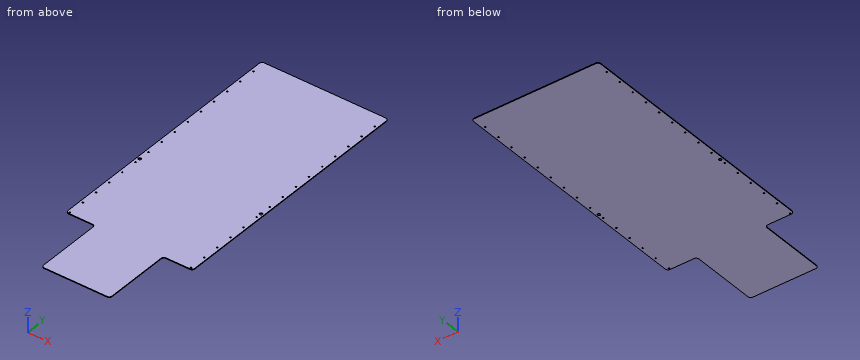
Autodesk Inventor part; units mm, degrees
ref_plane "YZ Plane" through (0, 0, 0) normal (1, 0, 0) x (0, 1, 0)
ref_plane "XZ Plane" through (0, 0, 0) normal (0, 1, 0) x (-1, 0, 0)
ref_plane "XY Plane" through (0, 0, 0) normal (0, 0, 1) x (1, 0, 0)
sketch "Sketch2" plane through (0, 0, 0) normal (0, 0, 1) x (1, 0, 0)
  line L0 (0, 0) -> (566.42, 0)
  line L1 (566.42, 0) -> (566.42, -1727.2)
  line L2 (566.42, -1727.2) -> (0, -1727.2)
  line L3 (0, -1727.2) -> (0, 0)
  dimension "d0" = 566.42
  dimension "d1" = 1727.2
extrude "Extrusion1" add sketch "Sketch2" along normal blind 3.175
sketch "Sketch4" plane through (0, 0, 3.175) normal (0, 0, 1) x (1, 0, 0)
  line L0 (566.42, 0) -> (0, 0)
  line L1 (0, 0) -> (0, -1727.2)
  line L2 (0, -1727.2) -> (566.42, -1727.2)
  line L3 (566.42, -1727.2) -> (566.42, 0)
  line L4 (0, -1727.2) -> (566.42, -1727.2)
  line L5 (68.58, -1727.2) -> (500.38, -1727.2)
  circle A0 centre (68.58, -1391.92) radius 12.7
  circle A1 centre (500.38, -1391.92) radius 12.7
  circle A2 centre (68.58, -1727.2) radius 12.7
  circle A3 centre (500.38, -1727.2) radius 12.7
  dimension "d6" = 25.4
  dimension "d7" = 25.4
  dimension "d8" = 25.4
  dimension "d9" = 25.4
extrude "Extrusion2" add sketch "Sketch4" along normal blind 3.175 contours A0 | A1
sketch "Sketch6" plane through (0, 0, 3.175) normal (0, 0, 1) x (1, 0, 0)
  circle A0 centre (12.7, -1460.5) radius 3.175
  circle A1 centre (553.72, -1460.5) radius 3.175
  circle A2 centre (553.72, -1460.5) radius 4.7625
  circle A3 centre (12.7, -1460.5) radius 4.7625
  point P0 (0, 0)
  dimension "d16" = 9.525
  dimension "d17" = 9.525
extrude "Extrusion4" cut sketch "Sketch6" against normal through all contours A0 | A1 | A2 | A3
sketch "Sketch7" plane through (0, 0, 3.175) normal (0, 0, 1) x (1, 0, 0)
  circle A0 centre (12.7, -1460.5) radius 4.7625
  circle A1 centre (12.7, -1460.5) radius 6.35
  circle A2 centre (553.72, -1460.5) radius 4.7625
  circle A3 centre (553.72, -1460.5) radius 6.35
  point P0 (0, 0)
  dimension "d20" = 12.7
  dimension "d21" = 12.7
extrude "Extrusion5" cut sketch "Sketch7" against normal blind 12.7 contours A3
sketch "Sketch9" plane through (0, 0, 3.175) normal (0, 0, 1) x (1, 0, 0)
  circle A0 centre (553.72, -825.5) radius 6.35
  circle A1 centre (12.7, -825.5) radius 6.35
  circle A2 centre (12.7, -825.5) radius 6.35
  circle A3 centre (553.72, -825.5) radius 6.35
  point P0 (0, 0)
extrude "Extrusion7" cut sketch "Sketch9" against normal blind 3.175
sketch "Sketch10" plane through (0, 0, 3.175) normal (0, 0, 1) x (1, 0, 0)
  line L0 (566.42, 0) -> (566.42, -1727.2)
  line L1 (0, -1732.8892) -> (566.42, -1732.8892)
  line L2 (566.42, -1732.8892) -> (566.42, -1054.0894)
  line L3 (566.42, -1054.0894) -> (0, -1054.0894)
  line L4 (0, -1054.0894) -> (0, -1732.8892)
  point P0 (0, 0)
extrude "Extrusion8" cut sketch "Sketch10" along normal blind 25.4
sketch "Sketch12" plane through (0, 0, 0) normal (0, 0, -1) x (-1, 0, 0)
  line L0 (-133.5248, -1752.8599) -> (-130.3498, -1752.8599)
  line L1 (-130.3498, -1752.8599) -> (-130.3498, -1726.7719)
  line L2 (-130.3498, -1726.7719) -> (-133.5248, -1726.7719)
  line L3 (-133.5248, -1726.7719) -> (-133.5248, -1752.8599)
  line L4 (-133.5248, -1752.8599) -> (-130.3498, -1752.8599)
  line L5 (-133.5248, -1777.5719) -> (-133.5248, -1752.8599)
  line L6 (-82.7248, -1777.5719) -> (-133.5248, -1777.5719)
  line L7 (-82.7248, -1774.3969) -> (-82.7248, -1777.5719)
  line L8 (-130.3498, -1774.3969) -> (-82.7248, -1774.3969)
  line L9 (-130.3498, -1752.8599) -> (-130.3498, -1774.3969)
  line L10 (-130.3498, -1237.6912) -> (0, -1237.6912)
  line L11 (0, -1237.6912) -> (0, -1727.2)
  line L12 (0, -1727.2) -> (-130.3498, -1727.2)
  line L13 (-130.3498, -1727.2) -> (-130.3498, -1237.6912)
  line L14 (0, -1727.2) -> (-566.42, -1727.2)
  line L15 (-566.8989, -1237.6912) -> (-436.5461, -1237.6912)
  line L16 (-436.5461, -1237.6912) -> (-436.5461, -1727.2)
  line L17 (-436.5461, -1727.2) -> (-566.8989, -1727.2)
  line L18 (-566.8989, -1727.2) -> (-566.8989, -1237.6912)
  point P0 (0, 0)
  point P1 (-108.1248, -1263.0912)
  dimension "d32" = 130.3528
extrude "Extrusion9" cut sketch "Sketch12" against normal blind 3.175 contours L1 L13 L10 L11 L12
sketch "Sketch13" plane through (0, 0, 0) normal (0, 0, -1) x (-1, 0, 0)
  line L0 (-566.42, -1727.2) -> (-566.42, 0)
  line L1 (-130.3498, -1727.2) -> (-566.42, -1727.2)
  line L2 (-566.42, -1239.5747) -> (-435.131, -1239.5747)
  line L3 (-435.131, -1239.5747) -> (-435.131, -1727.2)
  line L4 (-435.131, -1727.2) -> (-566.42, -1727.2)
  line L5 (-566.42, -1727.2) -> (-566.42, -1239.5747)
  point P0 (0, 0)
extrude "Extrusion10" cut sketch "Sketch13" against normal blind 3.175
sketch "Sketch14" plane through (0, 0, 0) normal (0, 0, -1) x (-1, 0, 0)
  line L0 (-130.3498, -1727.2) -> (-130.3498, -1237.6912)
  line L1 (-435.131, -1727.2) -> (-130.3498, -1727.2)
  line L2 (-130.3498, -1727.2) -> (-130.3498, -1549.4)
  line L3 (-130.3498, -1549.4) -> (-435.131, -1549.4)
  line L4 (-435.131, -1549.4) -> (-435.131, -1727.2)
  point P0 (0, 0)
  dimension "d35" = 177.8
extrude "Extrusion11" cut sketch "Sketch14" against normal blind 3.175
hole "Hole1" at (12.7, -12.7, 3.175) direction (0, 0, -1) diameter 6.35 depth 12.7 tip angle 118
pattern_linear "Rectangular Pattern1" count 17 spacing 76.2 along (0, -1, 0) of "Hole1"
hole "Hole2" at (553.72, -12.7, 3.175) direction (0, 0, -1) diameter 6.35 depth 12.7 tip angle 118
pattern_linear "Rectangular Pattern2" count 17 spacing 76.2 along (0, -1, 0) of "Hole2"
fillet "Fillet1" radius 12.7 8 edges at (566.42, 0, 1.5875) (0, 0, 1.5875) (566.42, -1239.5747, 1.5875) (435.131, -1239.5747, 1.5875) (435.131, -1549.4, 1.5875) (0, -1237.6912, 1.5875) (130.3498, -1237.6912, 1.5875) (130.3498, -1549.4, 1.5875)
sketch "Sketch15" plane through (0, 0, 3.175) normal (0, 0, 1) x (1, 0, 0)
  arc A0 (130.3498, -1536.7) -> (143.0498, -1549.4) centre (143.0498, -1536.7) ccw
  line L0 (143.0498, -1549.4) -> (422.431, -1549.4)
  arc A1 (422.431, -1549.4) -> (435.131, -1536.7) centre (422.431, -1536.7) ccw
  line L1 (435.131, -1536.7) -> (435.131, -1252.2747)
  arc A2 (447.831, -1239.5747) -> (435.131, -1252.2747) centre (447.831, -1252.2747) ccw
  line L2 (447.831, -1239.5747) -> (553.72, -1239.5747)
  arc A3 (553.72, -1239.5747) -> (566.42, -1226.8747) centre (553.72, -1226.8747) ccw
  line L3 (566.42, -1226.8747) -> (566.42, -12.7)
  arc A4 (566.42, -12.7) -> (553.72, 0) centre (553.72, -12.7) ccw
  line L4 (553.72, 0) -> (12.7, 0)
  arc A5 (12.7, 0) -> (0, -12.7) centre (12.7, -12.7) ccw
  line L5 (0, -12.7) -> (0, -1224.9912)
  arc A6 (0, -1224.9912) -> (12.7, -1237.6912) centre (12.7, -1224.9912) ccw
  line L6 (12.7, -1237.6912) -> (117.6498, -1237.6912)
  arc A7 (130.3498, -1250.3912) -> (117.6498, -1237.6912) centre (117.6498, -1250.3912) ccw
  line L7 (130.3498, -1250.3912) -> (130.3498, -1536.7)
  circle A8 centre (12.7, -825.5) radius 6.35
  circle A9 centre (553.72, -825.5) radius 6.35
  circle A10 centre (12.7, -12.7) radius 3.175
  circle A11 centre (12.7, -88.9) radius 3.175
  circle A12 centre (12.7, -165.1) radius 3.175
  circle A13 centre (12.7, -241.3) radius 3.175
  circle A14 centre (12.7, -317.5) radius 3.175
  circle A15 centre (12.7, -393.7) radius 3.175
  circle A16 centre (12.7, -469.9) radius 3.175
  circle A17 centre (12.7, -546.1) radius 3.175
  circle A18 centre (12.7, -622.3) radius 3.175
  circle A19 centre (12.7, -698.5) radius 3.175
  circle A20 centre (12.7, -774.7) radius 3.175
  circle A21 centre (12.7, -850.9) radius 3.175
  circle A22 centre (12.7, -927.1) radius 3.175
  circle A23 centre (12.7, -1003.3) radius 3.175
  circle A24 centre (12.7, -1079.5) radius 3.175
  circle A25 centre (12.7, -1155.7) radius 3.175
  circle A26 centre (12.7, -1231.9) radius 3.175
  circle A27 centre (553.72, -12.7) radius 3.175
  circle A28 centre (553.72, -88.9) radius 3.175
  circle A29 centre (553.72, -165.1) radius 3.175
  circle A30 centre (553.72, -241.3) radius 3.175
  circle A31 centre (553.72, -317.5) radius 3.175
  circle A32 centre (553.72, -393.7) radius 3.175
  circle A33 centre (553.72, -469.9) radius 3.175
  circle A34 centre (553.72, -546.1) radius 3.175
  circle A35 centre (553.72, -622.3) radius 3.175
  circle A36 centre (553.72, -698.5) radius 3.175
  circle A37 centre (553.72, -774.7) radius 3.175
  circle A38 centre (553.72, -850.9) radius 3.175
  circle A39 centre (553.72, -927.1) radius 3.175
  circle A40 centre (553.72, -1003.3) radius 3.175
  circle A41 centre (553.72, -1079.5) radius 3.175
  circle A42 centre (553.72, -1155.7) radius 3.175
  circle A43 centre (553.72, -1231.9) radius 3.175
  line L8 (0, 0) -> (566.42, 0)
  line L9 (566.42, 0) -> (566.42, -101.6)
  line L10 (566.42, -101.6) -> (0, -101.6)
  line L11 (0, -101.6) -> (0, 0)
  dimension "d63" = 101.6
extrude "Extrusion12" cut sketch "Sketch15" against normal blind 25.4 contours L5 A5 L4 A4 L3 L10 | L11 L8 A5 | A4 L8 L9
fillet "Fillet2" radius 12.7 1 edges at (566.42, -101.6, 1.5875)
fillet "Fillet3" radius 12.7 1 edges at (0, -101.6, 1.5875)
equation "\"d22\" = d20"
properties part number "Back plate"
CAD build for the part. Positions are in the model's coordinates, mm. Coordinates: 2 decimals unless noted, no trailing zeros. Loops run counter-clockwise (first coordinate to the right, second up) from the corner with the lowest first, then second, coordinate; pieces in that order, holes last. Notation, with made-up numbers: (20.25, 17.25) - (40.25, 17.25) arc R25 cw to (40.25, 40.25) - close; hole circle Ø10 at (-33.5, 4). An arc over 180 degrees is marked (long way). Write item = value, one per line. Start each with the question number.
Q1. Cut at B-B, the plane y = -1452. List the corners of the cut face in (x, z) (3 decimals), then the cut area to 3 significant figures.
Q2. Drill centre lines: L1, parallel to X at y = -241.3, z = 1.85 (3 decimals); L2, parallel to Y at x = 513.5, z = 1.9; L3, parallel to X at y = -1226, z = 0.7. Where is each one in solid material? Low to high.
Q3. Flat gauge pin, fed straight in: pin 1 Ø5.5 at (x, y) = (553.72, -622.3) entering from -Z. Where does the tip first touch, or does it go through?
Q4. Cut at A-A, the plane z = 0.8. Give the number of separate pieces and of enclosed holes in the cut face, then the cut area to 3 significant figures.
Computed:
q1.outline = (130.35, 0) - (435.131, 0) - (435.131, 3.175) - (130.35, 3.175) - close
q1.area = 968 mm²
q2.L1 = 0 to 9.525, 15.875 to 550.545, 556.895 to 566.42
q2.L2 = -1239.57 to -101.6
q2.L3 = 0.04 to 566.42
q3.pin_1 = through
q4.separate_pieces = 1
q4.enclosed_holes = 32
q4.area = 737,000 mm²
